```python
from build123d import *

# Parameters (mm, degrees)
CLAMP_START          = -20.15
CLAMP_X_COVER_DEPTH  = 37.1
EAR_START            = -26.1
SKETCH2_W            = 5.2
SKETCH2_H            = 2.45
EAR_X_COVER_26_DEPTH = 5.95
EAR_START_2          = 16.95
SKETCH3_W            = 5.2
SKETCH3_H            = 2.45
EAR_X_COVER_17_DEPTH = 5.95
CUT_EXTRUDE1_START   = 18.9
SKETCH4_R            = 1.1
CUT_EXTRUDE1_DEPTH   = 2.65
CUT_EXTRUDE2_START   = 18.99
SKETCH5_R            = 2
CUT_EXTRUDE2_DEPTH   = 1.22
BOSS_EXTRUDE4_START  = 7.69
SKETCH6_W            = 0.7
SKETCH6_H            = 1.5
BOSS_EXTRUDE4_DEPTH  = 11.11
BOSS_EXTRUDE5_START  = 7.69
SKETCH7_W            = 0.7
SKETCH7_H            = 1.5
BOSS_EXTRUDE5_DEPTH  = 11.11


with BuildPart() as part:
    # Sketch1 → Clamp -X cover (new body)
    with BuildSketch(Plane.XY.offset(CLAMP_START)):
        Polygon((-17.397275866, 18.8), (-13.367148847, 18.8), (-13.367148847, 26.696897507), (-17.397275866, 24.370102587), align=None)
    extrude(amount=CLAMP_X_COVER_DEPTH)

    # Sketch2 → Ear -X cover -26 (add)
    with BuildSketch(Plane.XY.offset(EAR_START)):
        with Locations((-15.35, 20.225)):
            Rectangle(SKETCH2_W, SKETCH2_H)
    extrude(amount=EAR_X_COVER_26_DEPTH)

    # Sketch3 → Ear -X cover 17 (add)
    with BuildSketch(Plane.XY.offset(EAR_START_2)):
        with Locations((-15.35, 20.225)):
            Rectangle(SKETCH3_W, SKETCH3_H)
    extrude(amount=EAR_X_COVER_17_DEPTH)

    # Sketch4 → Cut-Extrude1 (cut)
    with BuildSketch(Plane(origin=(0, 0, 0), x_dir=(1, 0, 0), z_dir=(0, 1, 0)).offset(CUT_EXTRUDE1_START)):
        with Locations(Location((-15.35, 23.2, 0), (0, 0, 90))):
            Circle(SKETCH4_R)
        with Locations(Location((-15.35, -20, 0), (0, 0, 90))):
            Circle(SKETCH4_R)
    extrude(amount=CUT_EXTRUDE1_DEPTH, mode=Mode.SUBTRACT)

    # Sketch5 → Cut-Extrude2 (cut)
    with BuildSketch(Plane(origin=(0, 0, 0), x_dir=(1, 0, 0), z_dir=(0, 1, 0)).offset(CUT_EXTRUDE2_START)):
        with Locations(Location((-15.35, 23.2, 0), (0, 0, 270))):
            Circle(SKETCH5_R)
        with Locations(Location((-15.35, -20, 0), (0, 0, 270))):
            Circle(SKETCH5_R)
    extrude(amount=CUT_EXTRUDE2_DEPTH, mode=Mode.SUBTRACT)

    # Sketch6 → Boss-Extrude4 (add)
    with BuildSketch(Plane(origin=(0, 0, 0), x_dir=(1, 0, 0), z_dir=(0, 1, 0)).offset(BOSS_EXTRUDE4_START)):
        with Locations((-17.6, 8)):
            Rectangle(SKETCH6_W, SKETCH6_H)
    extrude(amount=BOSS_EXTRUDE4_DEPTH)

    # Sketch7 → Boss-Extrude5 (add)
    with BuildSketch(Plane(origin=(0, 0, 0), x_dir=(1, 0, 0), z_dir=(0, 1, 0)).offset(BOSS_EXTRUDE5_START)):
        with Locations((-17.6, -12)):
            Rectangle(SKETCH7_W, SKETCH7_H)
    extrude(amount=BOSS_EXTRUDE5_DEPTH)


solid = part.part
```
CAD build for the part. Positions are in the model's coordinates, mm. A direction names the side the tool comes from. Round coordinates to 2 decimals unless told otherwise and drop trailing zeros. Loops run counter-clockwise (first coordinate to the right, second up) from the corner with the lowest first, then second, coordinate; pieces in that order, holes last. Notation, with made-up numbers: (14.5, 46) - (60.5, 46) arc R23 cw to (60.5, 62) - close; hole circle Ø6 at (-8.5, 57.25). An arc over 180 degrees is marked (long way). Return JSON: item names as keys, results as strings. Group by question number.
Q1. Band-saw the part on A-A on z = 20. Give the cut face in (x, y), plus the area to 3 significant figures.
Q2. Flat gauge pins, fed straight in: pin 1 Ø0.8 at (x, y) = (-17.5, 14.5) entering from +Z; pin 2 Ø1.6 at (x, z) = (-14.5, -22.5) entering from +Y; pin 3 Ø0.8 at (y, z) = (13.5, 12) entering from +X; pin 4 Ø3 at (x, z) = (-13.5, -6) entering from +Y. Where does each tip first touch, or does it go through?
Q3. Drill centre lines: line 1 along Z through (x, y) = (-15.35, 19.65); line 2 along X through (y, z) = (19.65, -23.2); line 3 along X through (y, z) = (20.95, 20). Where is each one in solid material? Low to high. Write a range as [from, to].
Q4. Band-saw the part on B-B on y = 18.25. Give the cut face in (x, z).
Q5. Band-saw the part on D-D on z = 12. Give the cut face in (x, y).
Q6. Tool access for faces 1 (the face through (-15, 19, -21)), 2 (the face through (-17.25, 13, 12)), 3 (the face through (-15, 24, 16.95)), 4 (the face through (-15, 24, -20.15)), 5 (the face through (-15.3, 20.21, 21.3)): list every direction of +Z, -Z, +X, -X, +Y, -Y with a clear straight run to the whole face (end or side of a thin tool).
Q7. Two-plate mould, pull along Z, no slides. Class faces 6 (the face through (-17.397, 22, -2)), 7 (the face through (-17.25, 13, -8)), 8 (the face through (-15, 20, 22.9)), 9 (the face through (-16.44, 20.82, -23.06)): +Z half, -Z half, draft (parallel to the pull), parting line (faces both ways), or undercut.
Q8. Band-saw the part on C-C on x = -15.35. Give the cut face in (y, z).
Solutions:
{
 "1": {"outline": "(-17.95, 19) - (-17.35, 19) - (-17.35, 20.21) - (-16.45, 20.21) - (-16.45, 21.45) - (-17.95, 21.45) - close; (-14.25, 20.21) - (-13.35, 20.21) - (-13.35, 19) - (-12.75, 19) - (-12.75, 21.45) - (-14.25, 21.45) - close", "area": "5.17 mm^2"},
 "2": {"pin 1": "stops at z = 12.75", "pin 2": "stops at y = 21.45", "pin 3": "stops at x = -17.25", "pin 4": "stops at y = 26.7"},
 "3": {"line 1": "z = [-26.1, -25.2], [-21.2, 18], [22, 22.9]", "line 2": "x = [-17.95, -17.35], [-13.35, -12.75]", "line 3": "x = [-17.95, -16.45], [-14.25, -12.75]"},
 "4": {"outline": "(-17.95, -8.75) - (-17.25, -8.75) - (-17.25, -7.25) - (-17.95, -7.25) - close; (-17.95, 11.25) - (-17.25, 11.25) - (-17.25, 12.75) - (-17.95, 12.75) - close"},
 "5": {"outline": "(-17.95, 7.69) - (-17.25, 7.69) - (-17.25, 18.8) - (-13.37, 18.8) - (-13.37, 26.7) - (-17.4, 24.37) - (-17.4, 18.8) - (-17.95, 18.8) - close"},
 "6": {"face 1": "-Z, +X, -X, -Y", "face 2": "+Z, -Z, +X, -Y", "face 3": "+Z, +X, -X, +Y", "face 4": "-Z, +X, -X, +Y", "face 5": "-Y"},
 "7": {"face 6": "undercut", "face 7": "draft", "face 8": "+Z half", "face 9": "undercut"},
 "8": {"outline": "(18.8, -20.15) - (19, -20.15) - (19, -21.2) - (20.21, -21.2) - (20.21, -22.1) - (21.45, -22.1) - (21.45, -20.15) - (25.55, -20.15) - (25.55, 16.95) - (21.45, 16.95) - (21.45, 18.9) - (20.21, 18.9) - (20.21, 18) - (19, 18) - (19, 16.95) - (18.8, 16.95) - close; (19, -26.1) - (21.45, -26.1) - (21.45, -24.3) - (20.21, -24.3) - (20.21, -25.2) - (19, -25.2) - close; (19, 22) - (20.21, 22) - (20.21, 21.1) - (21.45, 21.1) - (21.45, 22.9) - (19, 22.9) - close"}
}
